Part print with two shaded views. Sizes in mm from the minimum x, y, z corner. A direction names the side the tool comes from. Round coordinates to 2 decimals unless told otherwise and drop trailing zeros. Write each loop counter-clockwise with the first axis right and the second up, starting at its lowest first coordinate (ties: lowest second). Pieces come first, ordered by that corner, then holes. Notation, with made-up numbers: M -36,77.25 L -20,77.25 A32 ccw -20,105.25 Z; hole C 62.25,-27.5 d2. An arc over 180 degrees is marked long. Use one line per item in the form item = value. Start each with the question number.
Item 1: Cut at C-C, the plane y = 23.5. Give the cut face in (x, z), then the cut area to 3 significant figures.
Item 2: Cut at D-D, the plane x = 8. Give the cut face in (y, z), then the cut area to 3 significant figures.
Item 3: Cut at B-B, the plane z = 8.75. Give the cut face in (x, y), then the cut area to 3 significant figures.
Item 4: Probe L1, parallel to Y at x = 17, z = 9; L2, parallel to Z at x = 20.5, y = 26; L3, parallel to X at y = 25, z = 9.75. List the from-to ranges inside material, lowest first.
Item 5: Which spindle directions (+Z, -Z, +X, -X, +Y, -Y) get a long thin tool onto all of the face, cutting with end or side? Do the marked faces 1, 2 and 3. Say none if no direction does.
Item 6: Flat gauge pins, fed straight in: pin 1 Ø3 at (x, z) = (11, 1.5) entering from +Y; pin 2 Ø5 at (x, z) = (6, 4) entering from +Y; pin 3 Ø1 at (x, y) = (24.5, 12) entering from -Z. Where does each tip first touch, or does it go through?
Item 7: Mould opens along Y. For the marked faces 4, 5, 6 and 7 say: +Y half, -Y half, draft (parallel to the pull), parting line (faces both ways), or undercut.
Item 8: Cut at A-A, the plane x = 17. Give the cut face in (y, z), then the cut area to 3 significant figures.
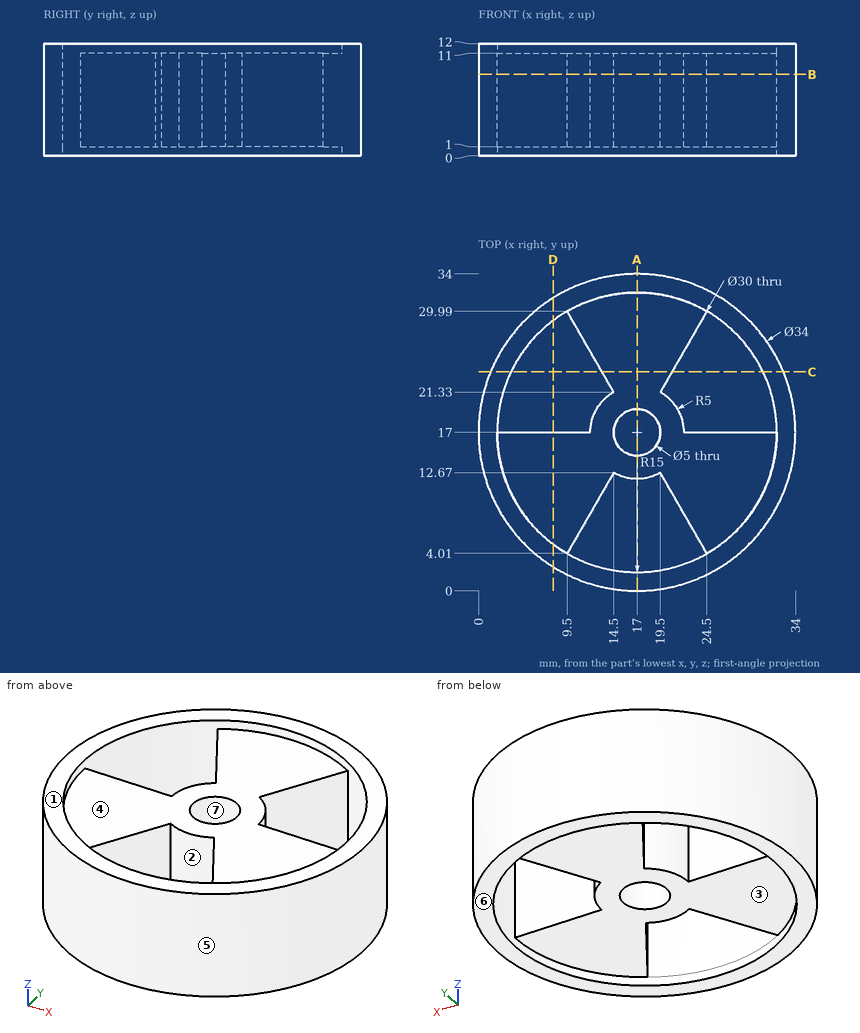
Model answer:
q1.outline = M 1.29,0 L 3.48,0 L 3.48,12 L 1.29,12 Z; M 13.25,1 L 20.75,1 L 20.75,11 L 13.25,11 Z; M 30.52,0 L 32.71,0 L 32.71,12 L 30.52,12 Z
q1.area = 128 mm²
q2.outline = M 2.58,0 L 5,0 L 5,1 L 17,1 L 17,11 L 5,11 L 5,12 L 2.58,12 Z; M 29,0 L 31.42,0 L 31.42,12 L 29,12 Z
q2.area = 178 mm²
q3.outline = C 17,17 d34; hole M 2,17 L 12,17 A5 cw 14.5,21.33 L 9.5,29.99 A15 ccw Z; hole M 9.5,4.01 A15 ccw 24.5,4.01 L 19.5,12.67 A5 cw 14.5,12.67 Z; hole C 17,17 d5; hole M 19.5,21.33 A5 cw 22,17 L 32,17 A15 ccw 24.5,29.99 Z
q3.area = 574 mm²
q4.L1 = 0 to 2, 12 to 14.5, 19.5 to 34
q4.L2 = 1 to 11
q4.L3 = 2 to 4.31, 12.38 to 21.62, 29.69 to 32
q5.face_1 = +Z, +X, -X, +Y, -Y
q5.face_2 = +Z, -Z
q5.face_3 = -Z
q6.pin_1 = 33.39
q6.pin_2 = 31.72
q6.pin_3 = 1
q7.face_4 = undercut
q7.face_5 = parting line
q7.face_6 = draft
q7.face_7 = undercut
q8.outline = M 0,0 L 2,0 L 2,12 L 0,12 Z; M 12,1 L 14.5,1 L 14.5,11 L 12,11 Z; M 19.5,1 L 32,1 L 32,0 L 34,0 L 34,12 L 32,12 L 32,11 L 19.5,11 Z
q8.area = 198 mm²
